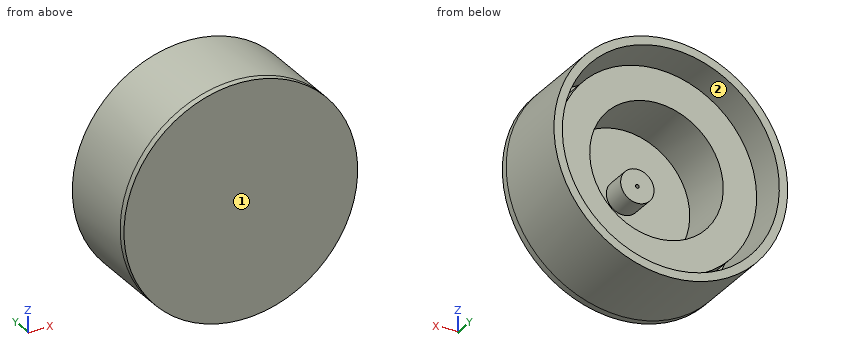
```python
from build123d import *

# Parameters (mm, degrees)
SKETCH1_R           = 70
SKETCH1_R_2         = 65
SKETCH1_R_3         = 60
SKETCH1_R_4         = 40
SKETCH1_R_5         = 10
SKETCH1_R_6         = 1.125
BOSS_EXTRUDE2_DEPTH = 4
SKETCH1_6_R         = 10
SKETCH1_6_R_2       = 1.125
BOSS_EXTRUDE3_DEPTH = 15
SKETCH1_7_R         = 70
SKETCH1_7_R_2       = 65
BOSS_EXTRUDE4_DEPTH = 50
SKETCH1_8_R         = 60
SKETCH1_8_R_2       = 40
BOSS_EXTRUDE5_DEPTH = 35


with BuildPart() as part:
    # Sketch1 → Boss-Extrude2 (new body)
    with BuildSketch(Plane(origin=(0, 0, 0), x_dir=(1, 0, 0), z_dir=(0, 1, 0))):
        with Locations(Location((0, 0, 0), (0, 0, 270))):
            Circle(SKETCH1_R)
        Circle(SKETCH1_R_2, mode=Mode.SUBTRACT)
        Circle(SKETCH1_R_2)
        Circle(SKETCH1_R_3, mode=Mode.SUBTRACT)
        Circle(SKETCH1_R_3)
        Circle(SKETCH1_R_4, mode=Mode.SUBTRACT)
        Circle(SKETCH1_R_4)
        Circle(SKETCH1_R_5, mode=Mode.SUBTRACT)
        Circle(SKETCH1_R_5)
        Circle(SKETCH1_R_6, mode=Mode.SUBTRACT)
        Circle(SKETCH1_R_6)
    extrude(amount=-BOSS_EXTRUDE2_DEPTH)

    # Sketch1_6 → Boss-Extrude3 (add)
    with BuildSketch(Plane(origin=(0, 0, 0), x_dir=(1, 0, 0), z_dir=(0, 1, 0))):
        with Locations(Location((0, 0, 0), (0, 0, 270))):
            Circle(SKETCH1_6_R)
        with Locations(Location((0, 0, 0), (0, 0, 270))):
            Circle(SKETCH1_6_R_2, mode=Mode.SUBTRACT)
    extrude(amount=BOSS_EXTRUDE3_DEPTH)

    # Sketch1_7 → Boss-Extrude4 (add)
    with BuildSketch(Plane(origin=(0, 0, 0), x_dir=(1, 0, 0), z_dir=(0, 1, 0))):
        with Locations(Location((0, 0, 0), (0, 0, 270))):
            Circle(SKETCH1_7_R)
        with Locations(Location((0, 0, 0), (0, 0, 270))):
            Circle(SKETCH1_7_R_2, mode=Mode.SUBTRACT)
    extrude(amount=BOSS_EXTRUDE4_DEPTH)

    # Sketch1_8 → Boss-Extrude5 (add)
    with BuildSketch(Plane(origin=(0, 0, 0), x_dir=(1, 0, 0), z_dir=(0, 1, 0))):
        with Locations(Location((0, 0, 0), (0, 0, 270))):
            Circle(SKETCH1_8_R)
        with Locations(Location((0, 0, 0), (0, 0, 270))):
            Circle(SKETCH1_8_R_2, mode=Mode.SUBTRACT)
    extrude(amount=BOSS_EXTRUDE5_DEPTH)


solid = part.part
```
Can you work these out from the model? Positions are in its coordinate system, mm. Face numbers are marked on the shaded views. Coordinates: 2 decimals unless noted, no trailing zeros. Loops run counter-clockwise (first coordinate to the right, second up) from the corner with the lowest first, then second, coordinate; pieces in that order, holes last. Notation, with made-up numbers: (-8, 75) -> (33, 75) arc R8 cw to (33, 85) -> close; hole circle Ø10 at (45.25, 82.5). An arc over 180 degrees is marked (long way). Answer as a JSON object with one key per item and string values.
1) For P1, Ø8, axis at x = 19, y = 23.5, coming from the +Z side; P2, Ø8, axis at x = -6, y = 5.5, coming from the -Z side; P3, Ø2, axis at x = -34, z = 26.5, coming from the +Y side, each with a flat end and sliding along its axis, tell me the tip position at first contact or that it passes through.
Results:
{"P1": "stops at z = 68.37", "P2": "stops at z = -69.97", "P3": "stops at y = 35"}
2) Imagine slicing it at D-D (x = 45). Please give me the cut outline in (y, z).
Results:
{"outline": "(-4, -53.62) -> (50, -53.62) -> (50, -46.9) -> (0, -46.9) -> (0, -39.69) -> (35, -39.69) -> (35, 39.69) -> (0, 39.69) -> (0, 46.9) -> (50, 46.9) -> (50, 53.62) -> (-4, 53.62) -> close"}
3) Thinking about a two-plate mould opening in Z: for the marked faces 1 and 2, which applies, pulls with the +Z half, pulls with the -Z half, needs draft (parallel to the pull), parting line crosses it, or undercut?
Results:
{"face 1": "needs draft", "face 2": "undercut"}
4) Imagine slicing it at A-A (y = 6). Please give me the cut outline in (x, z) (3 decimals).
Results:
{"outline": "circle Ø140 at (0, 0); circle Ø120 at (0, 0); circle Ø20 at (0, 0); hole circle Ø130 at (0, 0); hole circle Ø80 at (0, 0); hole circle Ø2.25 at (0, 0)"}
5) If I drill on line 1 (X direction, y = 26, z = 0); line 2 (X direction, y = 8, z = 35.5); line 3 (X direction, y = 13.5, z = 3.5), over which ranges is the centre line in solid material (lowest first)?
Results:
{"line 1": "x = -70 to -65, -60 to -40, 40 to 60, 65 to 70", "line 2": "x = -60.33 to -54.45, -48.37 to -18.43, 18.43 to 48.37, 54.45 to 60.33", "line 3": "x = -69.91 to -64.91, -59.9 to -39.85, -9.37 to 9.37, 39.85 to 59.9, 64.91 to 69.91"}
6) Imagine slicing it at C-C (z = -3). Please give me the cut outline in (x, y).
Results:
{"outline": "(-69.94, -4) -> (69.94, -4) -> (69.94, 50) -> (64.93, 50) -> (64.93, 0) -> (59.92, 0) -> (59.92, 35) -> (39.89, 35) -> (39.89, 0) -> (9.54, 0) -> (9.54, 15) -> (-9.54, 15) -> (-9.54, 0) -> (-39.89, 0) -> (-39.89, 35) -> (-59.92, 35) -> (-59.92, 0) -> (-64.93, 0) -> (-64.93, 50) -> (-69.94, 50) -> close"}
7) Imagine slicing it at B-B (y = 19.5). Please give me the cut outline in (x, z).
Results:
{"outline": "circle Ø140 at (0, 0); circle Ø120 at (0, 0); hole circle Ø130 at (0, 0); hole circle Ø80 at (0, 0)"}
